```python
from build123d import *

# Parameters (mm, degrees)
IZIM1_W                     = 25
IZIM1_H                     = 25
Y_KSEKLIK_EKSTR_ZYON1_DEPTH = 400
IZIM2_W                     = 20
IZIM2_H                     = 20
Y_KSEKLIK_EKSTR_ZYON2_DEPTH = 300
IZIM3_R                     = 5
Y_KSEKLIK_EKSTR_ZYON3_DEPTH = 5
IZIM4_W                     = 25
IZIM4_H                     = 2.554442859
Y_KSEKLIK_EKSTR_ZYON4_DEPTH = 15
RADYUS1_R                   = 10
IZIM6_R                     = 18.171292503
Y_KSEKLIK_EKSTR_ZYON5_DEPTH = 10
RADYUS2_R                   = 5
KES_EKSTR_ZYON2_DEPTH       = 58
IZIM8_R                     = 5
KES_EKSTR_ZYON3_DEPTH       = 32


with BuildPart() as part:
    # Çizim1 → Yükseklik-Ekstrüzyon1 (new body)
    with BuildSketch(Plane(origin=(0, 0, 0), x_dir=(1, 0, 0), z_dir=(0, 1, 0))):
        Rectangle(IZIM1_W, IZIM1_H)
    extrude(amount=Y_KSEKLIK_EKSTR_ZYON1_DEPTH)

    # Çizim2 → Yükseklik-Ekstrüzyon2 (add)
    with BuildSketch(Plane.XZ):
        Rectangle(IZIM2_W, IZIM2_H)
    extrude(amount=Y_KSEKLIK_EKSTR_ZYON2_DEPTH)

    # Çizim3 → Yükseklik-Ekstrüzyon3 (add)
    with BuildSketch(Plane.ZY.offset(12.5)):
        with Locations(Location((0, 20.234922869, 0), (0, 0, 180))):
            Circle(IZIM3_R)
    extrude(amount=Y_KSEKLIK_EKSTR_ZYON3_DEPTH)

    # Çizim4 → Yükseklik-Ekstrüzyon4 (add)
    with BuildSketch(Plane.ZY.offset(17.5)):
        with Locations((0, 20.23492287)):
            Rectangle(IZIM4_W, IZIM4_H)
    extrude(amount=Y_KSEKLIK_EKSTR_ZYON4_DEPTH)

    # Radyus1
    # the kernel refuses this fillet: 10 mm, written as the material it adds along each edge
    with BuildSketch(Plane(origin=(-17.5, 18.95770144, -29.834118888), x_dir=(0, -1, 0), z_dir=(0, 0, 1))) as radyus1_piece_1_section:
        with BuildLine():
            CenterArc((RADYUS1_R, -RADYUS1_R), RADYUS1_R, 90, 90)
            Line((0, -RADYUS1_R), (0, 0))
            Line((0, 0), (RADYUS1_R, 0))
        make_face()
    radyus1_piece_1 = extrude(amount=59.668237775, mode=Mode.PRIVATE)
    radyus1_piece_1 = radyus1_piece_1 & Plane(origin=(-20.338214919, 20.234922869, 0), x_dir=(0, 0, -1), z_dir=(1, 0, 0)) * Cylinder(5, 160, mode=Mode.PRIVATE)
    add(radyus1_piece_1)
    with BuildSketch(Plane(origin=(-17.5, 21.512144299, 29.834118888), x_dir=(0, 1, 0), z_dir=(0, 0, -1))) as radyus1_piece_2_section:
        with BuildLine():
            CenterArc((RADYUS1_R, -RADYUS1_R), RADYUS1_R, 90, 90)
            Line((0, -RADYUS1_R), (0, 0))
            Line((0, 0), (RADYUS1_R, 0))
        make_face()
    radyus1_piece_2 = extrude(amount=59.668237775, mode=Mode.PRIVATE)
    radyus1_piece_2 = radyus1_piece_2 & Plane(origin=(-20.33821492, 20.234922869, 0), x_dir=(0, 0, -1), z_dir=(1, 0, 0)) * Cylinder(5, 160, mode=Mode.PRIVATE)
    add(radyus1_piece_2)

    # Çizim6 → Yükseklik-Ekstrüzyon5 (add)
    with BuildSketch(Plane.XZ.offset(300)):
        with Locations(Location((0, 0, 0), (0, 0, 270))):
            Circle(IZIM6_R)
    extrude(amount=Y_KSEKLIK_EKSTR_ZYON5_DEPTH)

    # Radyus2
    # the kernel refuses this fillet: 5 mm, written as the material it adds along each edge
    with BuildSketch(Plane(origin=(10, -300, 10), x_dir=(1, 0, 0), z_dir=(0, 0, -1)), Plane(origin=(-10, -300, 10), x_dir=(0, 0, 1), z_dir=(1, 0, 0)), Plane(origin=(-10, -300, -10), x_dir=(-1, 0, 0), z_dir=(0, 0, 1)), Plane(origin=(10, -300, -10), x_dir=(0, 0, -1), z_dir=(-1, 0, 0))) as radyus2_piece_1:
        with BuildLine():
            CenterArc((RADYUS2_R, -RADYUS2_R), RADYUS2_R, 90, 90)
            Line((0, -RADYUS2_R), (0, 0))
            Line((0, 0), (RADYUS2_R, 0))
        make_face()
    extrude(amount=20)
    with BuildSketch(Plane(origin=(10, -300, 22.5), x_dir=(1, 0, 0), z_dir=(0, 0, -1))) as radyus2_piece_2a_section:
        with BuildLine():
            CenterArc((RADYUS2_R, -RADYUS2_R), RADYUS2_R, 90, 90)
            Line((0, -RADYUS2_R), (0, 0))
            Line((0, 0), (RADYUS2_R, 0))
        make_face()
    radyus2_piece_2a = extrude(amount=32.5, mode=Mode.PRIVATE)
    radyus2_piece_2a = radyus2_piece_2a & Plane(origin=(0, -298.735965494, 0), x_dir=(0, 0, -1), z_dir=(0, 1, 0)) * Cylinder(18.171292503, 85, mode=Mode.PRIVATE)
    radyus2_piece_2a = split(radyus2_piece_2a, bisect_by=Plane(origin=(10.899012229, -298.735965494, 10), z_dir=(0, 0, 1)), keep=Keep.TOP, mode=Mode.PRIVATE)
    with BuildSketch(Plane(origin=(-10, -300, 10), x_dir=(0, 0, 1), z_dir=(1, 0, 0))) as radyus2_piece_2b_section:
        with BuildLine():
            CenterArc((RADYUS2_R, -RADYUS2_R), RADYUS2_R, 90, 90)
            Line((0, -RADYUS2_R), (0, 0))
            Line((0, 0), (RADYUS2_R, 0))
        make_face()
    radyus2_piece_2b = extrude(amount=32.5, mode=Mode.PRIVATE)
    radyus2_piece_2b = radyus2_piece_2b & Plane(origin=(0, -298.73596552, 0), x_dir=(0, 0, -1), z_dir=(0, 1, 0)) * Cylinder(18.171292503, 85, mode=Mode.PRIVATE)
    radyus2_piece_2b = split(radyus2_piece_2b, bisect_by=Plane(origin=(10, -298.73596552, 10.899011766), z_dir=(1, 0, 0)), keep=Keep.TOP, mode=Mode.PRIVATE)
    radyus2_piece_2 = radyus2_piece_2a & radyus2_piece_2b
    add(radyus2_piece_2)
    with BuildSketch(Plane(origin=(22.5, -300, -10), x_dir=(0, 0, -1), z_dir=(-1, 0, 0))) as radyus2_piece_3a_section:
        with BuildLine():
            CenterArc((RADYUS2_R, -RADYUS2_R), RADYUS2_R, 90, 90)
            Line((0, -RADYUS2_R), (0, 0))
            Line((0, 0), (RADYUS2_R, 0))
        make_face()
    radyus2_piece_3a = extrude(amount=32.5, mode=Mode.PRIVATE)
    radyus2_piece_3a = radyus2_piece_3a & Plane(origin=(0, -298.735965494, 0), x_dir=(0, 0, -1), z_dir=(0, 1, 0)) * Cylinder(18.171292503, 85, mode=Mode.PRIVATE)
    radyus2_piece_3a = split(radyus2_piece_3a, bisect_by=Plane(origin=(10, -298.735965494, -10.899012229), z_dir=(1, 0, 0)), keep=Keep.TOP, mode=Mode.PRIVATE)
    with BuildSketch(Plane(origin=(10, -300, 10), x_dir=(1, 0, 0), z_dir=(0, 0, -1))) as radyus2_piece_3b_section:
        with BuildLine():
            CenterArc((RADYUS2_R, -RADYUS2_R), RADYUS2_R, 90, 90)
            Line((0, -RADYUS2_R), (0, 0))
            Line((0, 0), (RADYUS2_R, 0))
        make_face()
    radyus2_piece_3b = extrude(amount=32.5, mode=Mode.PRIVATE)
    radyus2_piece_3b = radyus2_piece_3b & Plane(origin=(0, -298.73596552, 0), x_dir=(0, 0, -1), z_dir=(0, 1, 0)) * Cylinder(18.171292503, 85, mode=Mode.PRIVATE)
    radyus2_piece_3b = split(radyus2_piece_3b, bisect_by=Plane(origin=(10.899011766, -298.73596552, -10), z_dir=(0, 0, -1)), keep=Keep.TOP, mode=Mode.PRIVATE)
    radyus2_piece_3 = radyus2_piece_3a & radyus2_piece_3b
    add(radyus2_piece_3)
    with BuildSketch(Plane(origin=(-22.5, -300, 10), x_dir=(0, 0, 1), z_dir=(1, 0, 0))) as radyus2_piece_4a_section:
        with BuildLine():
            CenterArc((RADYUS2_R, -RADYUS2_R), RADYUS2_R, 90, 90)
            Line((0, -RADYUS2_R), (0, 0))
            Line((0, 0), (RADYUS2_R, 0))
        make_face()
    radyus2_piece_4a = extrude(amount=32.5, mode=Mode.PRIVATE)
    radyus2_piece_4a = radyus2_piece_4a & Plane(origin=(0, -298.735965494, 0), x_dir=(0, 0, -1), z_dir=(0, 1, 0)) * Cylinder(18.171292503, 85, mode=Mode.PRIVATE)
    radyus2_piece_4a = split(radyus2_piece_4a, bisect_by=Plane(origin=(-10, -298.735965494, 10.899012229), z_dir=(-1, 0, 0)), keep=Keep.TOP, mode=Mode.PRIVATE)
    with BuildSketch(Plane(origin=(-10, -300, -10), x_dir=(-1, 0, 0), z_dir=(0, 0, 1))) as radyus2_piece_4b_section:
        with BuildLine():
            CenterArc((RADYUS2_R, -RADYUS2_R), RADYUS2_R, 90, 90)
            Line((0, -RADYUS2_R), (0, 0))
            Line((0, 0), (RADYUS2_R, 0))
        make_face()
    radyus2_piece_4b = extrude(amount=32.5, mode=Mode.PRIVATE)
    radyus2_piece_4b = radyus2_piece_4b & Plane(origin=(0, -298.73596552, 0), x_dir=(0, 0, -1), z_dir=(0, 1, 0)) * Cylinder(18.171292503, 85, mode=Mode.PRIVATE)
    radyus2_piece_4b = split(radyus2_piece_4b, bisect_by=Plane(origin=(-10.899011766, -298.73596552, 10), z_dir=(0, 0, 1)), keep=Keep.TOP, mode=Mode.PRIVATE)
    radyus2_piece_4 = radyus2_piece_4a & radyus2_piece_4b
    add(radyus2_piece_4)
    with BuildSketch(Plane(origin=(10, -300, -10), x_dir=(0, 0, -1), z_dir=(-1, 0, 0))) as radyus2_piece_5a_section:
        with BuildLine():
            CenterArc((RADYUS2_R, -RADYUS2_R), RADYUS2_R, 90, 90)
            Line((0, -RADYUS2_R), (0, 0))
            Line((0, 0), (RADYUS2_R, 0))
        make_face()
    radyus2_piece_5a = extrude(amount=32.5, mode=Mode.PRIVATE)
    radyus2_piece_5a = radyus2_piece_5a & Plane(origin=(0, -298.73596552, 0), x_dir=(0, 0, -1), z_dir=(0, 1, 0)) * Cylinder(18.171292503, 86, mode=Mode.PRIVATE)
    radyus2_piece_5a = split(radyus2_piece_5a, bisect_by=Plane(origin=(-10, -298.73596552, -10.899011766), z_dir=(-1, 0, 0)), keep=Keep.TOP, mode=Mode.PRIVATE)
    with BuildSketch(Plane(origin=(-10, -300, -22.5), x_dir=(-1, 0, 0), z_dir=(0, 0, 1))) as radyus2_piece_5b_section:
        with BuildLine():
            CenterArc((RADYUS2_R, -RADYUS2_R), RADYUS2_R, 90, 90)
            Line((0, -RADYUS2_R), (0, 0))
            Line((0, 0), (RADYUS2_R, 0))
        make_face()
    radyus2_piece_5b = extrude(amount=32.5, mode=Mode.PRIVATE)
    radyus2_piece_5b = radyus2_piece_5b & Plane(origin=(0, -298.735965494, 0), x_dir=(0, 0, -1), z_dir=(0, 1, 0)) * Cylinder(18.171292503, 85, mode=Mode.PRIVATE)
    radyus2_piece_5b = split(radyus2_piece_5b, bisect_by=Plane(origin=(-10.899012229, -298.735965494, -10), z_dir=(0, 0, -1)), keep=Keep.TOP, mode=Mode.PRIVATE)
    radyus2_piece_5 = radyus2_piece_5a & radyus2_piece_5b
    add(radyus2_piece_5)

    # Çizim7 → Kes-Ekstrüzyon2 (cut)
    with BuildSketch(Plane(origin=(0, 0, -12.5), x_dir=(-1, 0, 0), z_dir=(0, 0, -1))):
        Polygon((12.5, 400), (-29.263602087, 348.205056807), (-29.263602087, 417.124411345), (12.5, 417.124411345), align=None)
    extrude(amount=-KES_EKSTR_ZYON2_DEPTH, mode=Mode.SUBTRACT)

    # Çizim8 → Kes-Ekstrüzyon3 (cut)
    with BuildSketch(Plane(origin=(187.878801042, 151.491535729, 0), x_dir=(0, 0, -1), z_dir=(0.7784608732437974, 0.6276931326918469, 0))):
        with Locations(Location((0, 299.402134432, 0), (0, 0, 90))):
            Circle(IZIM8_R)
    extrude(amount=-KES_EKSTR_ZYON3_DEPTH, mode=Mode.SUBTRACT)


solid = part.part
```
The listing builds one solid part. Answer for the finished solid, in the listing's coordinates (mm). A direction names the side the tool comes from. Coordinates: 2 decimals unless noted, no trailing zeros. Loops run counter-clockwise (first coordinate to the right, second up) from the corner with the lowest first, then second, coordinate; pieces in that order, holes last. Notation, with made-up numbers: M 34,30.25 L 62,30.25 A19 cw 62,62.25 Z; hole C 74.25,46 d10. An arc over 180 degrees is marked long. Answer as a JSON object with one key per item and string values. Group by question number.
Item 1: Each of these flat-tipped pins is pushed along its axis until it touches: P1, Ø2, axis at x = -25.5, y = 19.5, coming from the -Z side; P2, Ø1, axis at x = 2, z = -17, coming from the +Y side; P3, Ø10, axis at y = 47, z = 9.5, coming from the -X side. Where does it stop, or does it pass through?
Item 2: Section A-A (y = -22) is taken. Write down the section's boundary in (x, z).
Item 3: Determine the mould class of faces 4 (the face through (-2.953, 388.16, -2.953)), 5 (the face through (0, -310, 0)), 6 (the face through (-10, -145, 0)), 7 (the face through (12.5, 182, 0)) for opening direction Y: +Y half, -Y half, draft (parallel to the pull), parting line (faces both ways), or undercut.
Item 4: Section B-B (y = 345) is taken. Write down the section's boundary in (x, z), and give its area (3 significant figures).
Item 5: Consider L1, parallel to X at y = -16, z = 3.5; L2, parallel to Y at x = -23.5, z = 11; L3, parallel to Y at x = -14.5, z = -3.5. Determine where each line is inside the solid, lowest interval first.
Item 6: Which of the six approach directions +Z, -Z, +X, -X, +Y, -Y give full straight-line access (tool end or side, diameter ignored) to faces 1 (the face through (0, -145, 10)), 2 (the face through (0, 197, -12.5)), 3 (the face through (0, 197, 12.5))?
Solved:
{
 "1": {"P1": "stops at z = -12.5", "P2": "stops at y = -300", "P3": "stops at x = -12.5"},
 "2": {"outline": "M -10,-10 L 10,-10 L 10,10 L -10,10 Z"},
 "3": {"face 4": "+Y half", "face 5": "-Y half", "face 6": "undercut", "face 7": "draft"},
 "4": {"outline": "M -12.5,-12.5 L 12.5,-12.5 L 12.5,12.5 L -12.5,12.5 Z", "area": "625 mm2"},
 "5": {"L1": "x = -10 to 10", "L2": "y = 18.96 to 21.51", "L3": "y = -310 to -299.97, 16.66 to 23.81"},
 "6": {"face 1": "+Z, +X, -X", "face 2": "-Z, +X, -X, +Y", "face 3": "+Z, +X, -X, +Y"}
}
